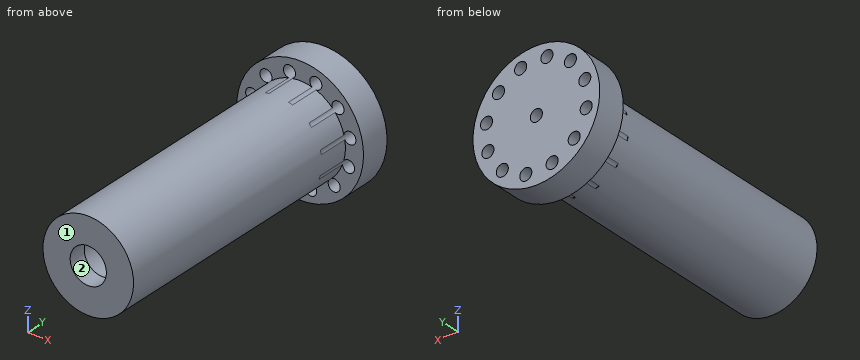
from build123d import *

# Parameters (mm, degrees)
SKETCH2_R          = 1
CUT_EXTRUDE1_DEPTH = 10
SKETCH3_R          = 3
CUT_EXTRUDE3_DEPTH = 10
SKETCH4_R          = 1
CUT_EXTRUDE4_DEPTH = 53.158412553


with BuildPart() as part:
    # Sketch1 → Revolve1 (revolve)
    with BuildSketch(Plane.XY, mode=Mode.PRIVATE) as revolve1_sk:
        Polygon((0, 0), (0, 3), (4.1, 3), (4.1, 18), (0, 18), (0, 50), (7.5, 50), (10.5, 50), (10.5, 45), (7.5, 45), (7.5, 0), align=None)
    revolve(revolve1_sk.sketch.rotate(Axis((0, 18, 0), (0, 1, 0)), 90), axis=Axis((0, 18, 0), (0, 1, 0)))

    # Sketch2 → Cut-Extrude1 (cut)
    with BuildSketch(Plane(origin=(0, 50, 0), x_dir=(1, 0, 0), z_dir=(0, 1, 0))):
        with Locations(Location((-2.60602925, 8.021687752, 0), (0, 0, 180))):
            Circle(SKETCH2_R)
        with Locations(Location((1.753956343, 8.25, 0), (0, 0, 180))):
            Circle(SKETCH2_R)
        with Locations(Location((5.64397075, 6.26773141, 0), (0, 0, 180))):
            Circle(SKETCH2_R)
        with Locations(Location((8.021687752, 2.60602925, 0), (0, 0, 180))):
            Circle(SKETCH2_R)
        with Locations(Location((8.25, -1.753956343, 0), (0, 0, 180))):
            Circle(SKETCH2_R)
        with Locations(Location((6.26773141, -5.64397075, 0), (0, 0, 180))):
            Circle(SKETCH2_R)
        with Locations(Location((2.60602925, -8.021687752, 0), (0, 0, 180))):
            Circle(SKETCH2_R)
        with Locations(Location((-1.753956343, -8.25, 0), (0, 0, 180))):
            Circle(SKETCH2_R)
        with Locations(Location((-5.64397075, -6.26773141, 0), (0, 0, 180))):
            Circle(SKETCH2_R)
        with Locations(Location((-8.021687752, -2.60602925, 0), (0, 0, 180))):
            Circle(SKETCH2_R)
        with Locations(Location((-8.25, 1.753956343, 0), (0, 0, 180))):
            Circle(SKETCH2_R)
        with Locations(Location((-6.26773141, 5.64397075, 0), (0, 0, 180))):
            Circle(SKETCH2_R)
    extrude(amount=-CUT_EXTRUDE1_DEPTH, mode=Mode.SUBTRACT)

    # Sketch3 → Cut-Extrude3 (cut)
    with BuildSketch(Plane.XZ):
        Circle(SKETCH3_R)
    extrude(amount=-CUT_EXTRUDE3_DEPTH, mode=Mode.SUBTRACT)

    # Sketch4 → Cut-Extrude4 (cut, through all)
    with BuildSketch(Plane(origin=(0, 50, 0), x_dir=(1, 0, 0), z_dir=(0, 1, 0))):
        with Locations(Location((0, 0, 0), (0, 0, 270))):
            Circle(SKETCH4_R)
    extrude(amount=-CUT_EXTRUDE4_DEPTH, mode=Mode.SUBTRACT)


solid = part.part
Part model, mm, in its own coordinate system. Face numbers are marked on the shaded views. A direction names the side the tool comes from. Round coordinates to 2 decimals unless told otherwise and drop trailing zeros. Order: outer loops, then holes, each group sorted by start corner. A loop starts at its lowest first (then second) coordinate and runs counter-clockwise, first axis right, second up. Notation, with made-up numbers: (55.5, -6.75) -> (101.5, -6.75) arc R24 cw to (101.5, 5.25) -> close; hole circle Ø11 at (-26.5, -4). An arc over 180 degrees is marked (long way). Put each result on its own line as item: value.
Q1. Band-saw the part on A-A (z = 0). Give the cut face in (x, y).
From the geometry:
outline: (-10.5, 45) -> (-7.5, 45) -> (-7.5, 0) -> (-3, 0) -> (-3, 3) -> (-4.1, 3) -> (-4.1, 18) -> (-1, 18) -> (-1, 50) -> (-10.5, 50) -> close; (1, 18) -> (4.1, 18) -> (4.1, 3) -> (3, 3) -> (3, 0) -> (7.5, 0) -> (7.5, 45) -> (10.5, 45) -> (10.5, 50) -> (1, 50) -> close
Q2. Band-saw the part on C-C (y = 12). Give the cut face in (x, z).
From the geometry:
outline: circle Ø15 at (0, 0); hole circle Ø8.2 at (0, 0)
Q3. Tool access for the marked faces 1 and 2: list every direction of +Z, -Z, +X, -X, +Y, -Y with a clear straight run to the whole face (end or side of a thin tool).
From the geometry:
face 1: +Z, -Z, +X, -X, -Y
face 2: -Y
Q4. Band-saw the part on B-B (x = 0). Give the cut face in (y, z).
From the geometry:
outline: (0, -7.5) -> (45, -7.5) -> (45, -10.5) -> (50, -10.5) -> (50, -1) -> (18, -1) -> (18, -4.1) -> (3, -4.1) -> (3, -3) -> (0, -3) -> close; (0, 3) -> (3, 3) -> (3, 4.1) -> (18, 4.1) -> (18, 1) -> (50, 1) -> (50, 10.5) -> (45, 10.5) -> (45, 7.5) -> (0, 7.5) -> close
Q5. Pin check, flat tips, straight feed: pin 1 Ø1.2 at (x, z) = (1.75, -8.25) entering from -Y; pin 2 Ø6 at (y, z) = (19.5, 3) entering from -X; pin 3 Ø1.5 at (x, y) = (5, 41) entering from +Z; pin 4 Ø4 at (x, y) = (-5, 30) entering from +Z. Stop position of each tip, or through.
From the geometry:
pin 1: passes through
pin 2: stops at x = -7.5
pin 3: stops at z = 6.18
pin 4: stops at z = 6.87
Q6. Wall check: line 1 (Y direction, x = -1.25, z = 3.25); line 2 (X direction, y = 42, z = 0); line 3 (X direction, y = 46.75, z = 8.25). Give the ranges that are in metal, low to high. Write a range as [from, to].
From the geometry:
line 1: y = [0, 3], [18, 50]
line 2: x = [-7.5, -1], [1, 7.5]
line 3: x = [-6.5, -2.75], [-0.75, 1.63], [3.58, 6.5]
Q7. Band-saw the part on D-D (x = -8.25). Give the cut face in (y, z).
From the geometry:
outline: (45, -6.5) -> (50, -6.5) -> (50, -2.75) -> (45, -2.75) -> close; (45, -0.75) -> (50, -0.75) -> (50, 1.63) -> (45, 1.63) -> close; (45, 3.58) -> (50, 3.58) -> (50, 6.5) -> (45, 6.5) -> close
